For this review, use the dimensioned drawing (mm, ordinates from the lowest corner) and the shaded views. A direction names the side the tool comes from. Coordinates: 2 decimals unless noted, no trailing zeros. Write each loop counter-clockwise with the first axis right and the second up, starting at its lowest first coordinate (ties: lowest second). Pieces come first, ordered by that corner, then holes. Notation, with made-up numbers: (41.25, 19) -> (87.25, 19) arc R16 cw to (87.25, 29) -> close; hole circle Ø6 at (40.5, 25). An arc over 180 degrees is marked (long way). Put each result on its own line as item: value. Start each with the question number.
Item 1: Consider section A-A on y = 2.25. Give the number of separate pieces and of enclosed holes in the cut face, and give its area (3 significant figures).
Item 2: Consider section B-B on z = 7.5. Give the boundary of the cut face in (x, y), and give its area (3 significant figures).
Item 3: Consider section D-D on z = 17. Give the boundary of the cut face in (x, y), and give its area (3 significant figures).
Item 4: Consider section C-C on x = 17. Give the boundary of the cut face in (y, z), and give its area (3 significant figures).
Item 5: Insertion check: P1, Ø5, axis at x = 105.5, z = 20.5, coming from the -Y side; P2, Ø1.2, axis at x = 56.5, z = 6.5, coming from the -Y side. Each pin has a flat end and moves straight along its axis. Give the tip position at first contact, or say it passes through.
Item 6: To check wall thickness, follow L1, parallel to X at y = 3, z = 11.5; L2, parallel to X at y = 2.75, z = 20.5; L3, parallel to Z at x = 50.5, y = 2.5. State the ranges of each line that lie inside material, in increasing order.
Item 7: The part is to be moulded in two halves that separate along X. For the marked faces 1, 2 and 3, say which applies: +X half, -X half, draft (parallel to the pull), parting line (faces both ways), or undercut.
Item 8: For the marked faces 4 and 5, list the 3-axis set-ups (+Z, -Z, +X, -X, +Y, -Y) from which the entire face can be reached by the end or side of a thin tool; tool diameter is ignored.
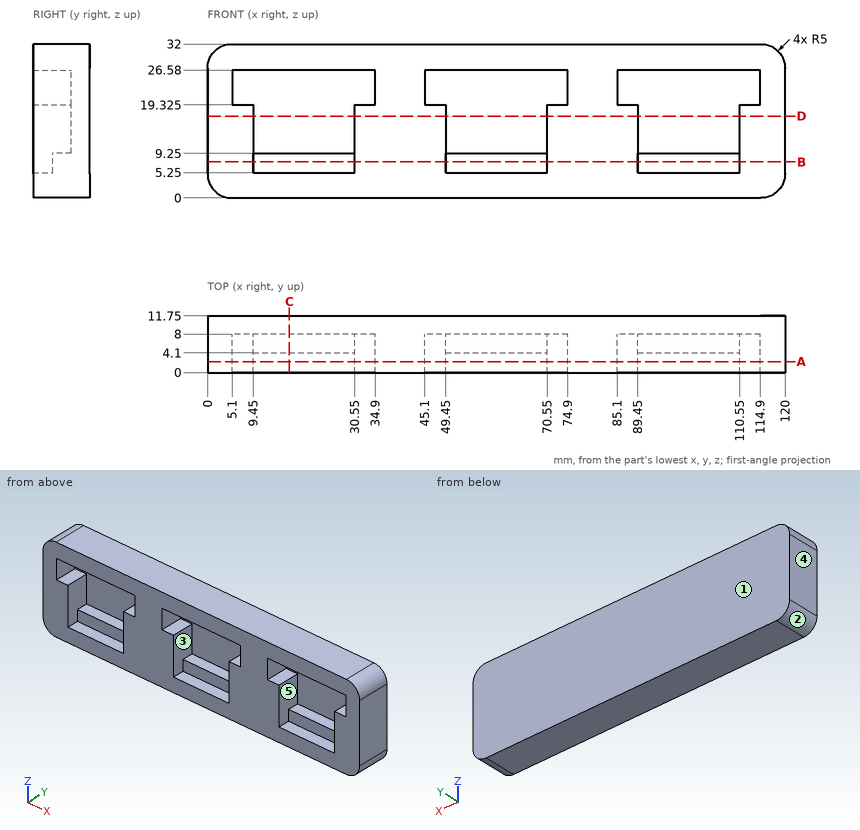
Return value:
1. separate pieces: 1
1. enclosed holes: 3
1. area: 2,280 mm^2
2. outline: (0, 0) -> (9.45, 0) -> (9.45, 4.1) -> (30.55, 4.1) -> (30.55, 0) -> (49.45, 0) -> (49.45, 4.1) -> (70.55, 4.1) -> (70.55, 0) -> (89.45, 0) -> (89.45, 4.1) -> (110.55, 4.1) -> (110.55, 0) -> (120, 0) -> (120, 11.75) -> (0, 11.75) -> close
2. area: 1,150 mm^2
3. outline: (0, 0) -> (9.45, 0) -> (9.45, 8) -> (30.55, 8) -> (30.55, 0) -> (49.45, 0) -> (49.45, 8) -> (70.55, 8) -> (70.55, 0) -> (89.45, 0) -> (89.45, 8) -> (110.55, 8) -> (110.55, 0) -> (120, 0) -> (120, 11.75) -> (0, 11.75) -> close
3. area: 904 mm^2
4. outline: (0, 0) -> (11.75, 0) -> (11.75, 32) -> (0, 32) -> (0, 26.58) -> (8, 26.58) -> (8, 9.25) -> (4.1, 9.25) -> (4.1, 5.25) -> (0, 5.25) -> close
4. area: 221 mm^2
5. P1: y = 8
5. P2: y = 4.1
6. L1: 0 to 9.45, 30.55 to 49.45, 70.55 to 89.45, 110.55 to 120
6. L2: 0 to 5.1, 34.9 to 45.1, 74.9 to 85.1, 114.9 to 120
6. L3: 0 to 5.25, 26.58 to 32
7. face 1: draft
7. face 2: -X half
7. face 3: undercut
8. face 4: +Z, -Z, -X, +Y, -Y
8. face 5: -Y
